The model under review builds one solid part; all positions refer to its coordinate system, in mm. Face numbers are marked on the shaded views. A direction names the side the tool comes from. Coordinates: 2 decimals unless noted, no trailing zeros. Loops run counter-clockwise (first coordinate to the right, second up) from the corner with the lowest first, then second, coordinate; pieces in that order, holes last. Notation, with made-up numbers: M 2.25,41 L 19.25,41 A24 ccw 19.25,66 Z; hole C -19.5,55 d9. An arc over 180 degrees is marked long. Return JSON: item names as keys, results as strings.
```python
from build123d import *

# Parameters (mm, degrees)
SKETCH1_W           = 2489.2
SKETCH1_H           = 1092.2
BOSS_EXTRUDE1_DEPTH = 889
SKETCH2_R           = 254
CUT_EXTRUDE1_DEPTH  = 50.8
SKETCH3_W           = 127
SKETCH3_H           = 127
BOSS_EXTRUDE2_DEPTH = 127


with BuildPart() as part:
    # Sketch1 → Boss-Extrude1 (new body)
    with BuildSketch(Plane(origin=(0, 0, 0), x_dir=(1, 0, 0), z_dir=(0, 1, 0))):
        Rectangle(SKETCH1_W, SKETCH1_H)
    extrude(amount=BOSS_EXTRUDE1_DEPTH)

    # Sketch2 → Cut-Extrude1 (cut)
    with BuildSketch(Plane.XY.offset(546.1)):
        with Locations((622.3, 444.5)):
            Circle(SKETCH2_R)
        with Locations((-622.3, 444.5)):
            Circle(SKETCH2_R)
    extrude(amount=-CUT_EXTRUDE1_DEPTH, mode=Mode.SUBTRACT)

    # Sketch3 → Boss-Extrude2 (add)
    with BuildSketch(Plane.XZ):
        with Locations((-1181.1, 482.6)):
            Rectangle(SKETCH3_W, SKETCH3_H)
        with Locations((-1181.1, -482.6)):
            Rectangle(SKETCH3_W, SKETCH3_H)
        with Locations((1181.1, 482.6)):
            Rectangle(SKETCH3_W, SKETCH3_H)
        with Locations((1181.1, -482.6)):
            Rectangle(SKETCH3_W, SKETCH3_H)
    extrude(amount=BOSS_EXTRUDE2_DEPTH)


solid = part.part
```
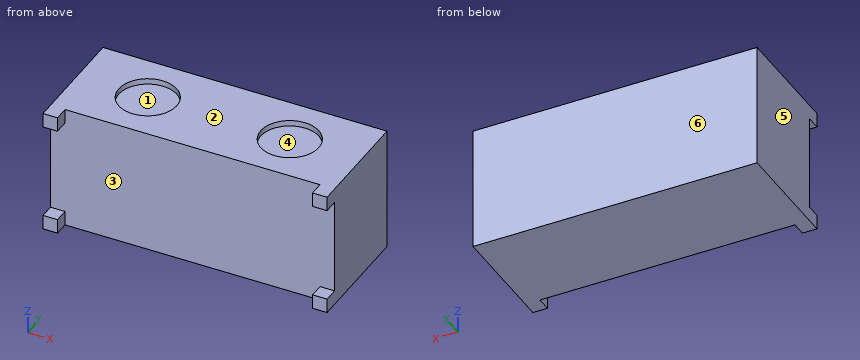
1. Machinability: for the marked faces 1 and 2, which of the approach directions +Z, -Z, +X, -X, +Y, -Y give a long, thin tool a straight path to every point of the face, cutting with its end or side? Answer none if there is none.
Check values:
{"face 1": "+Z", "face 2": "+Z, +X, -X, +Y, -Y"}
2. Insertion check: pin 1 Ø12 at (x, z) = (745.5, 54.5) entering from -Y. The pin has a flat end and moves straight along its axis. Give the tip position at first contact, or say it passes through.
Check values:
{"pin 1": "y = 0"}
3. Add section A-A on y = 444.5. Give the boundary of the cut face in (x, z), plus the area to 3 significant figures.
Check values:
{"outline": "M -1244.6,-546.1 L 1244.6,-546.1 L 1244.6,546.1 L 876.3,546.1 L 876.3,495.3 L 368.3,495.3 L 368.3,546.1 L -368.3,546.1 L -368.3,495.3 L -876.3,495.3 L -876.3,546.1 L -1244.6,546.1 Z", "area": "2,670,000 mm²"}
4. The part is to be moulded in two halves that separate along X. For the marked faces 3, 4, 5 and 6, say which applies: released by +X, released by -X, zero draft, split by the parting line, or undercut.
Check values:
{"face 3": "undercut", "face 4": "undercut", "face 5": "released by -X", "face 6": "zero draft"}
5. Add section C-C on z = 212. Give the boundary of the cut face in (x, y).
Check values:
{"outline": "M -1244.6,0 L 1244.6,0 L 1244.6,889 L -1244.6,889 Z"}
6. To check wall thickness, follow line 1 (X direction, y = 444, z = 522); line 2 (Y direction, x = 622, z = 508); line 3 (Y direction, x = 178, z = 163). State the ranges of each line that lie inside material, in increasing order.
Check values:
{"line 1": "-1244.6 to -876.3, -368.3 to 368.3, 876.3 to 1244.6", "line 2": "0 to 190.5, 698.5 to 889", "line 3": "0 to 889"}
7. Add section B-B on x = 622.3. Give the boundary of the cut face in (y, z).
Check values:
{"outline": "M 0,-546.1 L 889,-546.1 L 889,546.1 L 698.5,546.1 L 698.5,495.3 L 190.5,495.3 L 190.5,546.1 L 0,546.1 Z"}
8. Add section D-D on y = 595. Give the boundary of the cut face in (x, z).
Check values:
{"outline": "M -1244.6,-546.1 L 1244.6,-546.1 L 1244.6,546.1 L 826.91,546.1 L 826.91,495.3 L 417.69,495.3 L 417.69,546.1 L -417.69,546.1 L -417.69,495.3 L -826.91,495.3 L -826.91,546.1 L -1244.6,546.1 Z"}
